Read the model definition and answer for the solid it produces. Units are mm, in the model's axes. A direction names the side the tool comes from. Give positions to 0.01 mm unless a question says otherwise; leave off trailing zeros. Write each loop counter-clockwise with the first axis right and the second up, starting at its lowest first coordinate (ties: lowest second). Pieces come first, ordered by that corner, then holes. Notation, with made-up numbers: M -33,51 L -3,51 A17 ccw -3,55 Z; hole C -2.75,46 d7. An arc over 180 degrees is marked long. Put each result on its own line as item: value.
from build123d import *

# Parameters (mm, degrees)
SKETCH2_R           = 5
BOSS_EXTRUDE1_DEPTH = 8
FILLET1_R           = 1


with BuildPart() as part:
    # Sketch1 → Revolve1 (revolve)
    with BuildSketch(Plane.XY):
        with BuildLine():
            Line((-6.724338957, 69.005082459), (-12, 44.005082459))
            Line((-12, 44.005082459), (0, 44.005082459))
            Line((0, 44.005082459), (0, 77.950144306))
            ThreePointArc((0, 77.950144306), (-5.59532988, 75.156363932), (-6.724338957, 69.005082459))
        make_face()
    revolve(axis=Axis((0, 0, 0), (0, 1, 0)))

    # Sketch2 → Boss-Extrude1 (add)
    with BuildSketch(Plane.XZ.offset(-40.005082459)):
        Polygon((9.814954576, 0), (4.907477288, 8.5), (-4.907477288, 8.5), (-9.814954576, 0), (-4.907477288, -8.5), (4.907477288, -8.5), align=None)
        with Locations(Location((0, 0, 0), (0, 0, 270))):
            Circle(SKETCH2_R, mode=Mode.SUBTRACT)
    extrude(amount=-BOSS_EXTRUDE1_DEPTH)

    # Fillet1
    fillet1_edges = [part.edges().sort_by_distance(p)[0] for p in [
        (12, 44.005082459, 0),
    ]]
    fillet(fillet1_edges, radius=FILLET1_R)


solid = part.part
(1) For a pull along Z with two mould halves and no side action, classify faces 6 (the face through (-7.396, 41.977, -4.191)), 7 (the face through (7.396, 41.977, 4.191)), 8 (the face through (-4.88, 41.98, 1.08)) as +Z half, -Z half, draft (parallel to the pull), parting line (faces both ways), or undercut.
Result:
face 6: -Z half
face 7: +Z half
face 8: undercut
(2) Which of the six approach directions +Z, -Z, +X, -X, +Y, -Y give full straight-line access (tool end or side, diameter ignored) to faces 1 (the face through (0, 42, 8.5)), 2 (the face through (7.327, 41.977, -4.309)), 3 (the face through (0, 42, -8.5)), 4 (the face through (-7.327, 41.977, 4.309)), 5 (the face through (0, 44.005, 0))?
Result:
face 1: +Z, +X, -X, -Y
face 2: -Z, +X, -Y
face 3: -Z, +X, -X, -Y
face 4: +Z, -X, -Y
face 5: -Y
(3) Straight lines are drawn through the part: line 1 along X through (y, z) = (41.5, 0); line 2 along Z through (x, y) = (-5.25, 53.5); line 3 along Y through (x, z) = (-0.5, 5.75). For each, find the intervals that lie inside material, in ascending order. Write a range as from..to.
Result:
line 1: x = -9.81..-5, 5..9.81
line 2: z = -8.51..8.51
line 3: y = 40.01..74.91
(4) Section B-B on y = 64 is taken. Determine the outline of the cut face in (x, z).
Result:
outline: C 0,0 d15.56
(5) Section A-A on x = 0 is taken. Determine the outline of the cut face in (y, z), and give its area (3 significant figures).
Result:
outline: M 40.01,-8.5 L 44.01,-8.5 L 44.01,-10.77 A1 ccw 45.21,-11.75 L 69.01,-6.72 A7 ccw long 69.01,6.72 L 45.21,11.75 A1 ccw 44.01,10.77 L 44.01,8.5 L 40.01,8.5 L 40.01,5 L 44.01,5 L 44.01,-5 L 40.01,-5 Z
area: 599 mm²
(6) Section C-C on y = 58 is taken. Determine the outline of the cut face in (x, z), and give its area (3 significant figures).
Result:
outline: C 0,0 d18.09
area: 257 mm²
(7) Given pin 1 Ø8 at (y, z) = (71.5, 7) entering from -X; pin 2 Ø4 at (x, y) = (-1.5, 58) entering from -Z; pin 3 Ø11 at (x, z) = (-1, -1) entering from -Y; pin 4 Ø1 at (x, y) = (-7, 48) entering from +Z, each flat-ended and moving along its own axis, determine where each tip first touches the part or whether it passes through.
Result:
pin 1: stops at x = -6.31
pin 2: stops at z = -9.41
pin 3: stops at y = 40.01
pin 4: stops at z = 9.09
